Source: CAD feature listing. Evaluate the final solid. Frame: model axes, mm. Face numbers are marked on the shaded views. A direction names the side the tool comes from. Coordinates: 2 decimals unless noted, no trailing zeros. Order: outer loops, then holes, each group sorted by start corner. A loop starts at its lowest first (then second) coordinate and runs counter-clockwise, first axis right, second up. Notation, with made-up numbers: (39.5, -14.5) -> (68.5, -14.5) arc R25 cw to (68.5, 23.5) -> close; hole circle Ø4 at (20, -34). An arc over 180 degrees is marked (long way). Write item = value, one per line. Start each with the question number.
Item 1: Section query A-A (x = -2.5). Output: boundary loops of the cut face in (y, z), then the cut area to 3 significant figures.
Item 2: Section query D-D (y = 4.5). Output: boundary loops of the cut face in (x, z).
Item 3: Mould query, pull axis Z, two halves, no side actions, for the marked faces 4, 5 and 6. Classes: released by +Z, released by -Z, zero draft, split by the parting line, or undercut.
Item 4: Set-up query: the marked faces 1, 2 and 3. Return all of +Z, -Z, +X, -X, +Y, -Y with unobstructed straight access to the full face (end or side cutting, diameter ignored); none if empty.
Item 5: Ray query, line 1 along Y through (x, z) = (14.25, 6); line 2 along X through (y, z) = (6.8, 0); line 3 along Y through (x, z) = (-4, 1). Return the intervals inside material, ascending. Write a range as [from, to].
Item 6: Contact query for flat-ended pins moving along their axis: pin 1 (3.5 mm diameter, centred on y = 5, z = -6, fed in from +X); pin 2 (8 mm diameter, centred on x = -0.5, z = 2.5, fed in from +Y); pin 3 (4 mm diameter, centred on x = -10, z = -8, fed in from -Y); pin 4 (2 mm diameter, centred on y = 7.5, z = -4, fed in from -X). Output: stop coordinate, or through.
Item 7: Section query B-B (z = 0). Output: boundary loops of the cut face in (x, y).
Item 8: Section query C-C (y = 7.5). Output: boundary loops of the cut face in (x, z).
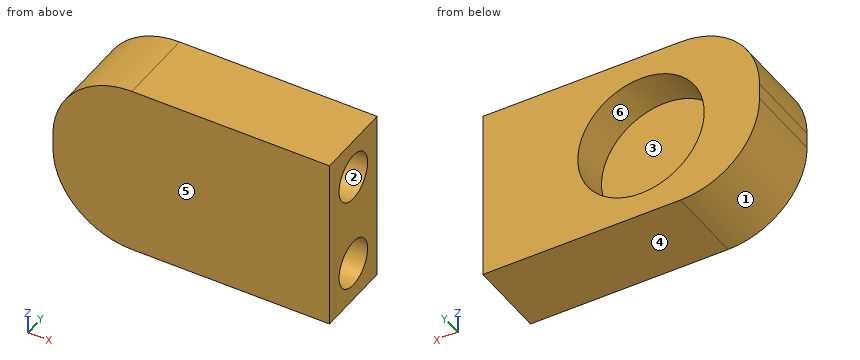
```python
from build123d import *

# Parameters (mm, degrees)
SKETCH1_W           = 35
SKETCH1_H           = 22
BOSS_EXTRUDE1_DEPTH = 10
SKETCH2_R           = 3
CUT_EXTRUDE1_DEPTH  = 10
SKETCH3_R           = 8
CUT_EXTRUDE2_DEPTH  = 5
FILLET1_R           = 10


with BuildPart() as part:
    # Sketch1 → Boss-Extrude1 (new body)
    with BuildSketch(Plane(origin=(0, 0, 0), x_dir=(1, 0, 0), z_dir=(0, 1, 0))):
        Rectangle(SKETCH1_W, SKETCH1_H)
    extrude(amount=BOSS_EXTRUDE1_DEPTH)

    # Sketch2 → Cut-Extrude1 (cut)
    with BuildSketch(Plane(origin=(17.5, 0, 0), x_dir=(0, 0, -1), z_dir=(1, 0, 0))):
        with Locations((6, 5)):
            Circle(SKETCH2_R)
        with Locations((-6, 5)):
            Circle(SKETCH2_R)
    extrude(amount=-CUT_EXTRUDE1_DEPTH, mode=Mode.SUBTRACT)

    # Sketch3 → Cut-Extrude2 (cut)
    with BuildSketch(Plane(origin=(0, 10, 0), x_dir=(1, 0, 0), z_dir=(0, 1, 0))):
        with Locations(Location((-2.5, 0, 0), (0, 0, 270))):
            Circle(SKETCH3_R)
    extrude(amount=-CUT_EXTRUDE2_DEPTH, mode=Mode.SUBTRACT)

    # Fillet1
    fillet1_edges = [part.edges().sort_by_distance(p)[0] for p in [
        (-17.5, 5, 11),
        (-17.5, 5, -11),
    ]]
    fillet(fillet1_edges, radius=FILLET1_R)


solid = part.part
```
Computed:
q1.outline = (0, -11) -> (10, -11) -> (10, -8) -> (5, -8) -> (5, 8) -> (10, 8) -> (10, 11) -> (0, 11) -> close
q1.area = 140 mm^2
q2.outline = (-17.5, -1) arc R10 ccw to (-7.5, -11) -> (17.5, -11) -> (17.5, -8.96) -> (7.5, -8.96) -> (7.5, -3.04) -> (17.5, -3.04) -> (17.5, 3.04) -> (7.5, 3.04) -> (7.5, 8.96) -> (17.5, 8.96) -> (17.5, 11) -> (-7.5, 11) arc R10 ccw to (-17.5, 1) -> close
q3.face_4 = released by -Z
q3.face_5 = zero draft
q3.face_6 = undercut
q4.face_1 = -Z, -X, +Y, -Y
q4.face_2 = +X
q4.face_3 = +Y
q5.line_1 = [0, 2], [8, 10]
q5.line_2 = [-17.5, -10.5], [5.5, 17.5]
q5.line_3 = [0, 5]
q6.pin_1 = 7.5
q6.pin_2 = 5
q6.pin_3 = 0
q6.pin_4 = -17.3
q7.outline = (-17.5, 0) -> (17.5, 0) -> (17.5, 10) -> (5.5, 10) -> (5.5, 5) -> (-10.5, 5) -> (-10.5, 10) -> (-17.5, 10) -> close
q8.outline = (-17.5, -1) arc R10 ccw to (-7.5, -11) -> (17.5, -11) -> (17.5, -7.66) -> (7.5, -7.66) -> (7.5, -4.34) -> (17.5, -4.34) -> (17.5, 4.34) -> (7.5, 4.34) -> (7.5, 7.66) -> (17.5, 7.66) -> (17.5, 11) -> (-7.5, 11) arc R10 ccw to (-17.5, 1) -> close; hole circle Ø16 at (-2.5, 0)
